from build123d import *

# Parameters (mm, degrees)
SKETCH1_W           = 67.400289577
SKETCH1_H           = 53.248033992
BOSS_EXTRUDE1_DEPTH = 2.54
LPATTERN1_COUNT     = 3
LPATTERN1_PITCH     = 12.7


with BuildPart() as part:
    # Sketch1 → Boss-Extrude1 (new body)
    with BuildSketch(Plane.XY):
        with Locations((-29.774643138, 13.689630717)):
            Rectangle(SKETCH1_W, SKETCH1_H)
    extrude(amount=BOSS_EXTRUDE1_DEPTH)

    # Sketch3 → CBORE for #2 Binding Head Machine Screw1 (revolve, cut)
    with BuildSketch(Plane(origin=(-30.833791182, 11.380076337, 2.54), x_dir=(0, -1, 0), z_dir=(1, 0, 0))):
        Polygon((0, 0), (0, 2.54), (1.1303, 2.54), (1.1303, 1.27), (2.77876, 1.27), (2.77876, 0.635), (3.41376, 0), align=None)
    cbore_for_2_binding_head_machine_screw1 = revolve(axis=Axis((-30.833791182, 11.380076337, 8.89), (0, 0, -1)), mode=Mode.SUBTRACT)

    # LPattern1: CBORE for #2 Binding Head Machine Screw1 ×3
    with Locations(*[(i * LPATTERN1_PITCH, 0, 0) for i in range(1, LPATTERN1_COUNT)]):
        add(cbore_for_2_binding_head_machine_screw1, mode=Mode.SUBTRACT)

    # Mirror1: CBORE for #2 Binding Head Machine Screw1 across plane
    add(cbore_for_2_binding_head_machine_screw1.mirror(Plane.ZX), mode=Mode.SUBTRACT)

    # Mirror1 copy 1 sketch → Mirror1 copy 1 (revolve, cut)
    with BuildSketch(Plane(origin=(-18.133791182, -11.380076337, 2.54), x_dir=(0, 1, 0), z_dir=(1, 0, 0))):
        Polygon((0, 0), (0, -2.54), (1.1303, -2.54), (1.1303, -1.27), (2.77876, -1.27), (2.77876, -0.635), (3.41376, 0), align=None)
    revolve(axis=Axis((-18.133791182, -11.380076337, 8.89), (0, 0, 1)), mode=Mode.SUBTRACT)

    # Mirror1 copy 2 sketch → Mirror1 copy 2 (revolve, cut)
    with BuildSketch(Plane(origin=(-5.433791182, -11.380076337, 2.54), x_dir=(0, 1, 0), z_dir=(1, 0, 0))):
        Polygon((0, 0), (0, -2.54), (1.1303, -2.54), (1.1303, -1.27), (2.77876, -1.27), (2.77876, -0.635), (3.41376, 0), align=None)
    revolve(axis=Axis((-5.433791182, -11.380076337, 8.89), (0, 0, 1)), mode=Mode.SUBTRACT)


solid = part.part
Model file for the job. Use its own axes, mm. A direction names the side the tool comes from. Give positions to 0.01 mm unless a question says otherwise; leave off trailing zeros. Write item = value, one per line.
Q1. Tool access for faces 1 (the flat face through (-18, -10, 1.27)), 2 (the flat face through (-30, 40.314, 1)): list every direction of +Z, -Z, +X, -X, +Y, -Y with a clear straight run to the whole face (end or side of a thin tool).
Derived:
face_1 = +Z
face_2 = +Z, -Z, +X, -X, +Y
Q2. Flat gauge pins, fed straight in: pin 1 (4.5 mm diameter, centred on x = -31, y = 12.5, fed in from +Z); pin 2 (2 mm diameter, centred on x = -31, y = -10, fed in from +Z); pin 3 (3.5 mm diameter, centred on x = -17, y = -11, fed in from +Z). Where does each tip first touch, or does it go through?
Derived:
pin_1 = 2.51
pin_2 = 1.27
pin_3 = 2.07
Q3. Two-plate mould, pull along X, no slides. Class faces 3 (the flat face through (3.926, 13, 1)), 4 (the cylindrical face through (-30.75, -8.603, 1.592)), 5 (the flat face through (-63.475, 13, 1)): pulls with the +X half, pulls with the -X half, needs draft (parallel to the pull), parting line crosses it, or undercut.
Derived:
face_3 = pulls with the +X half
face_4 = undercut
face_5 = pulls with the -X half
Q4. Drill centre lines: line 1 (X direction, y = 11.5, z = 0.6); line 2 (X direction, y = -9, z = 1.6). Where is each one in solid material? Low to high. Write a range as [from, to].
Derived:
line_1 = [-63.47, -31.96], [-29.71, -19.26], [-17.01, -6.56], [-4.31, 3.93]
line_2 = [-63.47, -32.27], [-29.4, -19.57], [-16.7, -6.87], [-4, 3.93]
